```python
from build123d import *

# Parameters (mm, degrees)
F1_DEPTH = 10
F2_R     = 11
F3_DEPTH = 10.001
F4_R     = 1


with BuildPart() as f1:
    # F0 (on Top) → F1 (new body)
    with BuildSketch(Plane.XY):
        with BuildLine():
            ThreePointArc((32.257237, -1.376276), (18.829424, 10.871173), (14.936729, 28.623724))
            ThreePointArc((14.936729, 28.623724), (0, 45), (-14.936729, 28.623724))
            ThreePointArc((-14.936729, 28.623724), (-18.829424, 10.871173), (-32.257237, -1.376276))
            ThreePointArc((-32.257237, -1.376276), (-38.971143, -22.5), (-17.320508, -27.247449))
            ThreePointArc((-17.320508, -27.247449), (0, -21.742346), (17.320508, -27.247449))
            ThreePointArc((17.320508, -27.247449), (38.971143, -22.5), (32.257237, -1.376276))
        make_face()
    extrude(amount=F1_DEPTH)

    # F2 (on face) → F3 (cut, through all)
    with BuildSketch(Plane.XY.offset(10)):
        with Locations((-25.980762, -15)):
            Circle(F2_R)
        Circle(F2_R)
        with Locations((0, 30)):
            Circle(F2_R)
        with Locations((25.980762, -15)):
            Circle(F2_R)
    extrude(amount=-F3_DEPTH, mode=Mode.SUBTRACT)

    # F4
    f4_edges = [f1.edges().sort_by_distance(p)[0] for p in [
        (0, -21.742346, 10),
    ]]
    fillet(f4_edges, radius=F4_R)


solid = f1.part
```
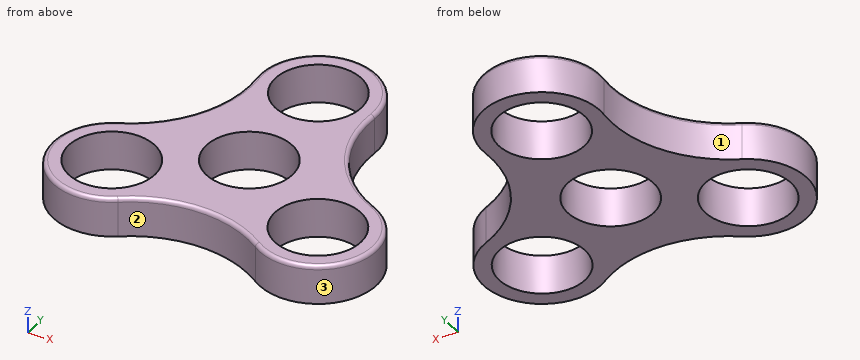
Geometry check sheet. Reference: the model listing, model coordinates, mm. Face numbers are marked on the shaded views. Round coordinates to 2 decimals unless told otherwise and drop trailing zeros. Loops run counter-clockwise (first coordinate to the right, second up) from the corner with the lowest first, then second, coordinate; pieces in that order, holes last. Notation, with made-up numbers: M -17,0.5 L -12,0.5 A11 ccw -12,11.5 Z; hole C -4,75.5 d6. An arc over 180 degrees is marked long. Return JSON: item names as keys, results as strings. Group by question number.
(1) Go/stop test with flat-tipped pins: pin 1 (4 mm diameter, centred on y = 4, z = 9, fed in from +X); pin 2 (5 mm diameter, centred on y = 22, z = 2, fed in from -X); pin 3 (1 mm diameter, centred on y = 14.5, z = 5.5, fed in from +X). Record where each tip stops, or that it passes through.
(2) Section check B-B, the plane z = 1.5. Enter the section's corners in (x, y), and give its area (3 significant figures).
(3) Section check A-A, the plane x = 0. Enter the section's corners in (y, z).
(4) Scan lines: line 1 along X through (y, z) = (-21.5, 9.25); line 2 along Y through (x, z) = (-1, 5.25); line 3 along Y through (x, z) = (-4, 8.75). Record each from-to range of solid material in increasing order. Write a range as [from, to].
(5) Section check C-C, the plane y = -15. Give the number of separate pieces and of enclosed holes in the cut face, and give its area (3 significant figures).
(6) Mould release check, pull along Y, two halves, no side actions. Record for the marked faces 1, 2 and 3: pulls with the +Y half, pulls with the -Y half, needs draft (parallel to the pull), parting line crosses it, or undercut.
Data:
{
 "1": {"pin 1": "x = 26.64", "pin 2": "x = -15.49", "pin 3": "x = 17.26"},
 "2": {"outline": "M -32.26,-1.38 A15 ccw long -17.32,-27.25 A30 cw 17.32,-27.25 A15 ccw long 32.26,-1.38 A30 cw 14.94,28.62 A15 ccw long -14.94,28.62 A30 cw Z; hole C -25.98,-15 d22; hole C 0,0 d22; hole C 0,30 d22; hole C 25.98,-15 d22", "area": "1,970 mm²"},
 "3": {"outline": "M -21.74,0 L -11,0 L -11,10 L -20.74,10 A1 ccw -21.74,9 Z; M 11,0 L 19,0 L 19,10 L 11,10 Z; M 41,0 L 45,0 L 45,9 A1 ccw 44,10 L 41,10 Z"},
 "4": {"line 1": "[-39.46, -34.85], [-17.11, 17.11], [34.85, 39.46]", "line 2": "[-21.76, -10.95], [10.95, 19.05], [40.95, 44.97]", "line 3": "[-22.01, -10.25], [10.25, 19.75], [40.25, 44.46]"},
 "5": {"separate pieces": "3", "enclosed holes": "0", "area": "379 mm²"},
 "6": {"face 1": "undercut", "face 2": "pulls with the -Y half", "face 3": "parting line crosses it"}
}
